```python
from build123d import *

# Parameters (mm, degrees)
F0_W                 = 118.4436753392
F0_H                 = 118.8980340958
F1_DEPTH             = 101.854
F4_D                 = 11.50874
F4_CSINK_D           = 23.8252
F4_CSINK_ANGLE       = 82
F4_ON_F2_D           = 11.50874
F4_ON_F2_CSINK_D     = 23.8252
F4_ON_F2_CSINK_ANGLE = 82


with BuildPart() as f1:
    # F0 (on Front) → F1 (new body)
    with BuildSketch(Plane.XZ):
        Rectangle(F0_W, F0_H)
    extrude(amount=F1_DEPTH)

    # F4 (through all)
    with Locations(Plane(origin=(-59.2218376696, 0, 0), x_dir=(0, -1, 0), z_dir=(-1, 0, 0))):
        with Locations((50.927, 0)):
            CounterSinkHole(F4_D / 2, F4_CSINK_D / 2, counter_sink_angle=F4_CSINK_ANGLE)

    # F4 on F2 (through all)
    with Locations(Plane.XY.offset(59.4490170479)):
        with Locations((0, -50.927)):
            CounterSinkHole(F4_ON_F2_D / 2, F4_ON_F2_CSINK_D / 2, counter_sink_angle=F4_ON_F2_CSINK_ANGLE)


solid = f1.part
```
Work out the finished part from the listing and answer in its coordinate system (mm). Give positions to 0.01 mm unless a question says otherwise; leave off trailing zeros. One line per item, written item: value. Start each with the question number.
1. Section A-A, the plane y = -48 is taken. Count the separate pieces of the cut face and the enclosed holes in it, then the cut area to 3 significant figures.
2. For a pull along Y with two mould halves and no side action, classify faces 1 (the face through (5.75, -50.67, 25.82)), 2 (the face through (-1, -101.854, 1)), 3 (the face through (-1, 0, 1)) as released by +Y, released by -Y, zero draft, split by the parting line, or undercut.
3. This flat-tipped pin is pushed along its axis until it touches: pin 1 Ø7 at (y, z) = (-50.927, 0) entering from -X. Where does it stop, or does it pass through?
4. Consider line 1 (Y direction, x = 0, z = -29.5); line 2 (Z direction, x = 22.5, y = -47); line 3 (Y direction, x = 3, z = 54). Determine where each line is inside the solid, lowest interval first.
Filled sheet:
1. separate pieces: 4
1. enclosed holes: 0
1. area: 11,700 mm²
2. face 1: undercut
2. face 2: released by -Y
2. face 3: released by +Y
3. pin 1: through
4. line 1: -101.85 to -56.68, -45.17 to 0
4. line 2: -59.45 to -4.21, 4.21 to 59.45
4. line 3: -101.85 to -57.45, -44.41 to 0
